```python
from build123d import *

# Parameters (mm, degrees)
SKETCH010_R          = 2.45
PAD007_DEPTH         = 1.6
PAD008_DEPTH         = 1.6
SKETCH059_W          = 3.1771358599
SKETCH059_H          = 6.2
POCKET022_DEPTH      = 1.6
POCKET022_DEPTH_BACK = 1.6


with BuildPart() as part:
    # Sketch010 → Pad007 (new body)
    with BuildSketch(Plane.YZ.offset(-8.7)):
        with BuildLine():
            ThreePointArc((-6, 6), (-7.4371881489, -9.1), (-6, -24.2))
            Line((-6, -24.2), (0, -24.2))
            ThreePointArc((0, -24.2), (4.2426406871, -22.4426406871), (6, -18.2))
            Line((6, 0), (6, -18.2))
            ThreePointArc((6, 0), (4.2426406871, 4.2426406871), (0, 6))
            Line((-6, 6), (0, 6))
        make_face()
        Circle(SKETCH010_R, mode=Mode.SUBTRACT)
        with Locations((0, -18.2)):
            Circle(SKETCH010_R, mode=Mode.SUBTRACT)
    extrude(amount=PAD007_DEPTH)

    # Sketch011 → Pad008 (join)
    with BuildSketch(Plane.YZ.offset(-8.7)):
        with BuildLine():
            ThreePointArc((5.8114989668, -16.707860677), (3.6774423219, -13.4590699257), (0, -12.2))
            Line((-7.3771358599, -12.2), (0, -12.2))
            ThreePointArc((-7.3771358599, -6), (-7.4371881489, -9.1), (-7.3771358599, -12.2))
            Line((-7.3771358599, -6), (0, -6))
            ThreePointArc((0, -6), (3.6774423219, -4.7409300743), (5.8114989668, -1.492139323))
            Line((5.8114989668, -1.492139323), (6, -0.7579762707))
            Line((6, -0.7579762707), (6, -17.4420237293))
            Line((6, -17.4420237293), (5.8114989668, -16.707860677))
        make_face()
    extrude(amount=-PAD008_DEPTH)

    # Sketch059 → Pocket022 (cut, two sides)
    with BuildSketch(Plane.YZ.offset(-8.7)) as pocket022_sk:
        with BuildLine():
            Line((-2.6, 6), (-2.6, 4.2))
            Line((-2.6, 4.2), (-6.3244944235, 4.2))
            ThreePointArc((-6, 6), (-6.167388681, 5.1009268767), (-6.3244944235, 4.2))
            Line((-6, 6), (-2.6, 6))
        make_face()
        with BuildLine():
            Line((-6, -24.2), (-2.6, -24.2))
            Line((-2.6, -24.2), (-2.6, -22.4))
            Line((-2.6, -22.4), (-6.3244944235, -22.4))
            ThreePointArc((-6.3244944235, -22.4), (-6.167388681, -23.3009268767), (-6, -24.2))
        make_face()
        with Locations((-4.18856793, -9.1)):
            Rectangle(SKETCH059_W, SKETCH059_H)
    extrude(amount=-POCKET022_DEPTH, mode=Mode.SUBTRACT)
    extrude(pocket022_sk.sketch, amount=POCKET022_DEPTH_BACK, mode=Mode.SUBTRACT)


with BuildPart() as part_1:
    # Body007 placement: moved
    add(part.part.moved(Location((0, -72.6064407756, 0))))


solid = part_1.part
```
Design review of the part built by this model. Coordinates are the model's own, in mm. A direction names the side the tool comes from. Round coordinates to 2 decimals unless told otherwise and drop trailing zeros. Order: outer loops, then holes, each group sorted by start corner. A loop starts at its lowest first (then second) coordinate and runs counter-clockwise, first axis right, second up. Notation, with made-up numbers: M 30,26 L 43,26 A12 cw 43,33 Z; hole C 34,55.5 d4. An arc over 180 degrees is marked long. Put each result on its own line as item: value.
Q1. Machinability: for faces 4 (the face through (-10.3, -70, -9)), 5 (the face through (-9.49, -68.89, -13.49)), 6 (the face through (-8, -77, -12.2)), 7 (the face through (-8, -75.206, -23)), 8 (the face through (-9, -74, -6)), which of the approach directions +Z, -Z, +X, -X, +Y, -Y give a long, thin tool a straight path to every point of the face, cutting with its end or side? Answer none if there is none.
Reported:
face 4: +Z, -Z, -X, +Y, -Y
face 5: -Z, -X, -Y
face 6: +X, -X
face 7: -Z, +X, -X, -Y
face 8: +Z, -X, -Y
Q2. To check wall thickness, follow line 1 (Y direction, x = -8.45, z = -10); line 2 (Z direction, x = -7.4, y = -70.75); line 3 (X direction, y = -77.75, z = 3). State the ranges of each line that lie inside material, in increasing order.
Reported:
line 1: -80.04 to -78.38, -75.21 to -66.61
line 2: -23.91 to -19.8, -16.6 to -1.6, 1.6 to 5.71
line 3: -8.7 to -7.1
Q3. Consider section A-A (y = -76.25). State the section outline as (x, z) points, and give its area (3 significant figures).
Reported:
outline: M -8.7,-22.4 L -7.1,-22.4 L -7.1,-12.2 L -8.7,-12.2 Z; M -8.7,-6 L -7.1,-6 L -7.1,4.2 L -8.7,4.2 Z
area: 32.6 mm²
Q4. Consider section D-D (y = -67.25). State the section outline as (x, z) points, and give its area (3 significant figures).
Reported:
outline: M -10.3,-15.5 L -8.7,-15.5 L -8.7,-20.9 L -7.1,-20.9 L -7.1,2.7 L -8.7,2.7 L -8.7,-2.7 L -10.3,-2.7 Z
area: 58.2 mm²
Q5. Consider section B-B (x = -8.1). State the section outline as (y, z) points, and give its area (3 significant figures).
Reported:
outline: M -78.93,-22.4 L -75.21,-22.4 L -75.21,-24.2 L -72.61,-24.2 A6 ccw -66.61,-18.2 L -66.61,0 A6 ccw -72.61,6 L -75.21,6 L -75.21,4.2 L -78.93,4.2 A80.04 ccw Z; hole M -78.38,-12.2 L -75.21,-12.2 L -75.21,-6 L -78.38,-6 Z; hole C -72.61,-18.2 d4.9; hole C -72.61,0 d4.9
area: 306 mm²
Q6. Insertion check: pin 1 Ø6 at (y, z) = (-76, -15.5) entering from -X; pin 2 Ø1.3 at (x, y) = (-9.5, -74) entering from +Z; pin 3 Ø1.5 at (x, y) = (-7.5, -71.5) entering from +Z. Each pin has a flat end and moves straight along its axis. Give the tip position at first contact, or say it passes through.
Reported:
pin 1: x = -8.7
pin 2: z = -6
pin 3: z = 5.99
Q7. Consider section C-C (y = -70.5). State the section outline as (x, z) points.
Reported:
outline: M -10.3,-12.58 L -8.7,-12.58 L -8.7,-16.95 L -7.1,-16.95 L -7.1,-1.25 L -8.7,-1.25 L -8.7,-5.62 L -10.3,-5.62 Z; M -8.7,-23.82 L -7.1,-23.82 L -7.1,-19.45 L -8.7,-19.45 Z; M -8.7,1.25 L -7.1,1.25 L -7.1,5.62 L -8.7,5.62 Z
Q8. Draft analysis for pull direction Z (two halves, no side actions). For faces 1 (the face through (-8, -77, -6)), 2 (the face through (-8, -77, -22.4)), 3 (the face through (-10.3, -79, -9)), state which applies: released by +Z, released by -Z, zero draft, split by the parting line, or undercut.
Reported:
face 1: undercut
face 2: released by -Z
face 3: zero draft
